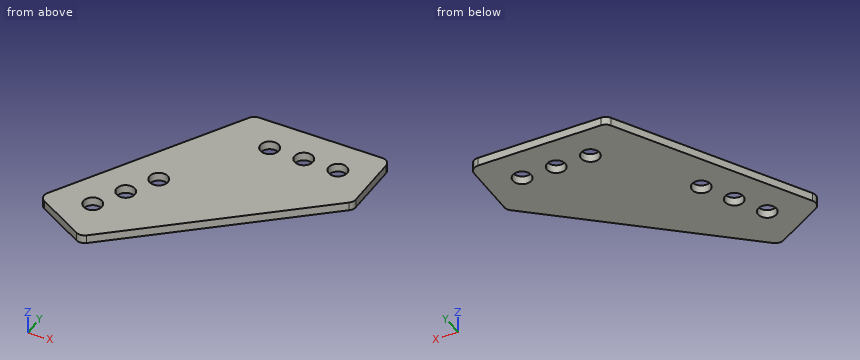
from build123d import *

# Parameters (mm, degrees)
SKETCH1_R           = 3.429
BOSS_EXTRUDE1_DEPTH = 3.175
FILLET1_R           = 3.175


with BuildPart() as part:
    # Sketch1 → Boss-Extrude1 (new body)
    with BuildSketch(Plane.XY):
        Polygon((0, 0), (50.8, 0), (50.8, -25.4), (-19.277954744, -84.190397082), (-41.275, -71.490397082), align=None)
        with Locations((38.1, -12.7)):
            Circle(SKETCH1_R, mode=Mode.SUBTRACT)
        with Locations((25.4, -12.7)):
            Circle(SKETCH1_R, mode=Mode.SUBTRACT)
        with Locations((12.7, -12.7)):
            Circle(SKETCH1_R, mode=Mode.SUBTRACT)
        with Locations((-23.926477372, -66.841874454)):
            Circle(SKETCH1_R, mode=Mode.SUBTRACT)
        with Locations((-17.576477372, -55.843351826)):
            Circle(SKETCH1_R, mode=Mode.SUBTRACT)
        with Locations((-11.226477372, -44.844829198)):
            Circle(SKETCH1_R, mode=Mode.SUBTRACT)
    extrude(amount=BOSS_EXTRUDE1_DEPTH)

    # Fillet1
    fillet1_edges = [part.edges().sort_by_distance(p)[0] for p in [
        (0, 0, 1.5875),
        (50.8, 0, 1.5875),
        (50.8, -25.4, 1.5875),
        (-19.277954744, -84.190397082, 1.5875),
        (-41.275, -71.490397082, 1.5875),
    ]]
    fillet(fillet1_edges, radius=FILLET1_R)


solid = part.part
Source: CAD feature listing. Evaluate the final solid. Frame: model axes, mm. Round coordinates to 2 decimals unless told otherwise and drop trailing zeros. Write each loop counter-clockwise with the first axis right and the second up, starting at its lowest first coordinate (ties: lowest second). Pieces come first, ordered by that corner, then holes. Notation, with made-up numbers: (-36, 47) - (-14, 47) arc R25 ccw to (-14, 64) - close; hole circle Ø1 at (3.25, 75). An arc over 180 degrees is marked (long way). Use CSV: the item, a comma, the result in double quotes. Start each with the question number.
(1) Material intervals for probe 1 along X at (y, z) = (-12, 1.25); probe 2 along Y at (x, z) = (25.5, 2.4); probe 3 along X at (y, z) = (-43.5, 2.55), sorted ascending. Write a range as [from, to].
(2) Cut plane B-B, the plane y = -12.7. Return loops of the section in (x, z) (3 decimals).
(3) Cut plane A-A, the plane x = 39. Return loops of the section in (y, z) (3 decimals), and give its area (3 significant figures).
(4) First-contact query: pin 1 Ø1.5 at (y, z) = (-74, 0.5) entering from -X; pin 2 Ø9 at (x, y) = (38.1, -12.7) entering from +Z (3 decimals). Flat tips, straight axial feed; report the tip coordinate or a pass-through.
(5) Cut plane C-C, the plane z = 0.65. Give the number of separate pieces and of enclosed holes in the cut face, and give its area (3 significant figures).
(6) Cut plane D-D, the plane y = -54. Return loops of the section in (x, z) (3 decimals).
Geometry says:
1,probe 1,"[-6.93, 9.34], [16.06, 22.04], [28.76, 34.74], [41.46, 50.8]"
1,probe 2,"[-46.62, -16.13], [-9.27, 0]"
1,probe 3,"[-25.11, -14.38], [-8.07, 29.22]"
2,outline,"(-7.332, 0) - (9.271, 0) - (9.271, 3.175) - (-7.332, 3.175) - close; (16.129, 0) - (21.971, 0) - (21.971, 3.175) - (16.129, 3.175) - close; (28.829, 0) - (34.671, 0) - (34.671, 3.175) - (28.829, 3.175) - close; (41.529, 0) - (50.8, 0) - (50.8, 3.175) - (41.529, 3.175) - close"
3,outline,"(-35.299, 0) - (-16.009, 0) - (-16.009, 3.175) - (-35.299, 3.175) - close; (-9.391, 0) - (0, 0) - (0, 3.175) - (-9.391, 3.175) - close"
3,area,"91.1 mm²"
4,pin 1,"x = -38.23"
4,pin 2,"z = 3.175"
5,separate pieces,"1"
5,enclosed holes,"6"
5,area,"3,850 mm²"
6,outline,"(-31.177, 0) - (-20.468, 0) - (-20.468, 3.175) - (-31.177, 3.175) - close; (-14.685, 0) - (16.709, 0) - (16.709, 3.175) - (-14.685, 3.175) - close"
